Geometry: final body of the model. Coordinates: model frame, mm. A direction names the side the tool comes from. Give positions to 0.01 mm unless a question says otherwise; leave off trailing zeros. Write each loop counter-clockwise with the first axis right and the second up, starting at its lowest first coordinate (ties: lowest second). Pieces come first, ordered by that corner, then holes.
Solid Edge part; units mm, degrees
sketch "Sketch1" plane through (0, 0, 0) normal (0, 0, 1) x (1, 0, 0)
  circle A0 centre (0, 0) radius 17.5
extrude "Protrusion1" add sketch "Sketch1" along normal blind 2
sketch "Sketch2" plane through (0, 0, 2) normal (0, 0, 1) x (1, 0, 0)
  line L0 (-5, 17.5) -> (5, 17.5)
  line L1 (5, 17.5) -> (5, -17.5)
  line L2 (5, -17.5) -> (-5, -17.5)
  line L3 (-5, -17.5) -> (-5, 17.5)
  dimension "D1" = 5
extrude "Extrusionsausschnitt_2" cut sketch "Sketch2" against normal blind 1
hole "Bohrung_1" at (0, 10, 0) direction (0, 0, 1) diameter 2 end up to next
pattern_linear "Pattern1" count 2 spacing 20 along (0, -1, 0) of "Bohrung_1"
properties part number "DV4" material "Polypropylen, hochfest"
Q1. Section D-D on y = 1.5. Output: boundary loops of the cut face in (x, z), plus the area to 3 significant figures.
Filled sheet:
outline: (-17.44, 0) - (17.44, 0) - (17.44, 2) - (5, 2) - (5, 1) - (-5, 1) - (-5, 2) - (-17.44, 2) - close
area: 59.7 mm2
Q2. Section B-B on z = 1.55. Output: boundary loops of the cut face in (x, y), plus the area to 3 significant figures.
Filled sheet:
outline: (-5, -16.77) - (-5, 16.77) arc R17.5 ccw to start; (5, -16.77) arc R17.5 ccw to (5, 16.77) - close
area: 617 mm2
Q3. Section A-A on x = 0. Output: boundary loops of the cut face in (y, z), plus the area to 3 significant figures.
Filled sheet:
outline: (-17.5, 0) - (-11, 0) - (-11, 1) - (-17.5, 1) - close; (-9, 0) - (9, 0) - (9, 1) - (-9, 1) - close; (11, 0) - (17.5, 0) - (17.5, 1) - (11, 1) - close
area: 31.0 mm2
Q4. Section C-C on y = 10. Output: boundary loops of the cut face in (x, z).
Filled sheet:
outline: (-14.36, 0) - (-1, 0) - (-1, 1) - (-5, 1) - (-5, 2) - (-14.36, 2) - close; (1, 0) - (14.36, 0) - (14.36, 2) - (5, 2) - (5, 1) - (1, 1) - close
Q5. Pull-direction query (Y, two-part tool) for faces 3 (the cylindrical face through (16.69, -5.26, 0.99)), 4 (the cylindrical face through (-0.6, -10.8, 0.5)), 5 (the flat face through (-5, -0.2, 1.5)), 6 (the cylindrical face through (-0.6, 9.2, 0.5)); classes: released by +Y, released by -Y, zero draft, split by the parting line, or undercut.
Filled sheet:
face 3: split by the parting line
face 4: undercut
face 5: zero draft
face 6: undercut
Q6. Pin query (flat end, axial travel): P1, Ø1.1, axis at y = 1.5, z = 1.5, coming from the +X side; P2, Ø1, axis at y = -9.5, z = 1.5, coming from the -X side; P3, Ø11, axis at x = -2, y = 0.5, coming from the +Z side; P4, Ø1, axis at y = -13.5, z = 1.5, coming from the -X side. Return the tip coordinate at first contact, or that it passes through.
Filled sheet:
P1: stops at x = 17.47
P2: stops at x = -15.01
P3: stops at z = 2
P4: stops at x = -11.72
Q7. Access query for faces 1 (the flat face through (0, 0, 1)), 2 (the flat face through (0, 0, 0)). Directions: +Z, -Z, +X, -X, +Y, -Y. A direction counts if a zero-diameter tool reaches every point of the face in a straight line with its end or side. Return the directions, or none.
Filled sheet:
face 1: +Z, +Y, -Y
face 2: -Z, +X, -X, +Y, -Y
Q8. Ray query, line 1 along Y through (x, z) = (0, 0.4); line 2 along Z through (x, y) = (4.5, 8); line 3 along X through (y, z) = (-10, 0.8). Return the intervals inside material, ascending.
Filled sheet:
line 1: y = -17.5 to -11, -9 to 9, 11 to 17.5
line 2: z = 0 to 1
line 3: x = -14.36 to -1, 1 to 14.36
